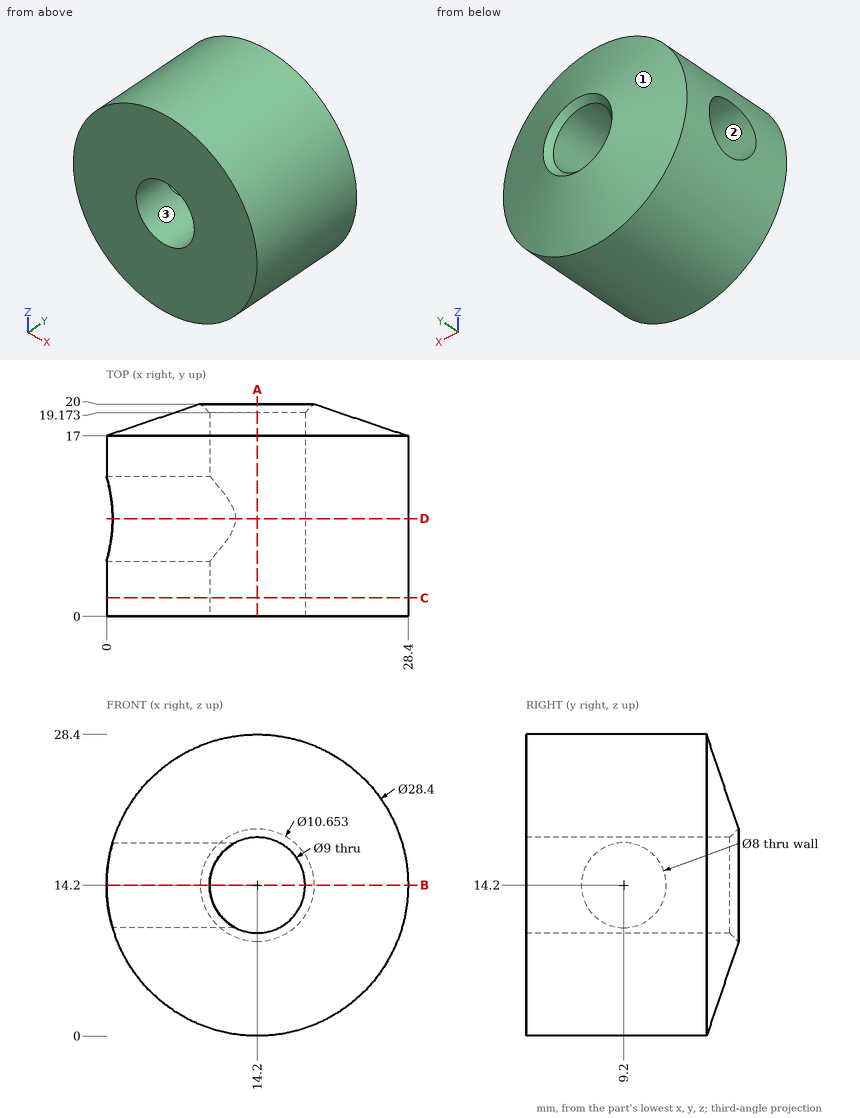
The figure shows three views and two pictorial views of one solid part (mm, origin at its lowest corner). Answer the questions. Round coordinates to 2 decimals unless told otherwise and drop trailing zeros. Write each loop counter-clockwise with the first axis right and the second up, starting at its lowest first coordinate (ties: lowest second). Pieces come first, ordered by that corner, then holes. Notation, with made-up numbers: (-8.75, 16) - (29.25, 16) arc R20 ccw to (29.25, 30) - close; hole circle Ø4 at (83, -24). An arc over 180 degrees is marked (long way). Use one line per item in the form item = value. Start each with the question number.
Item 1: Flat-ended cylindrical pins translate along their axes: pin 1 Ø10 at (y, z) = (8.5, 17.5) entering from -X; pin 2 Ø6 at (x, y) = (17.5, 6.5) entering from +Z; pin 3 Ø1 at (x, y) = (8.5, 2.5) entering from +Z; pin 4 Ø5 at (x, y) = (22, 17.5) entering from -Z. Find the tip coordinate at first contact, or state that the pin passes through.
Item 2: A cutting plane is placed at B-B (z = 14.2). Write down the section's boundary in (x, y).
Item 3: Find the intervals of material crossed by line 1 (X direction, y = 9.25, z = 14.2); line 2 (Z direction, x = 7.5, y = 8.5); line 3 (X direction, y = 14.25, z = 14.2), in increasing order. Write a range as [from, to].
Item 4: Determine the mould class of the marked faces 1, 2 and 3 for opening direction Y: +Y half, -Y half, draft (parallel to the pull), parting line (faces both ways), or undercut.
Item 5: A cutting plane is placed at D-D (y = 9.2). Write down the section's boundary in (x, z) (1 decimal).
Item 6: A cutting plane is placed at A-A (x = 14.2). Write down the section's boundary in (y, z), plus the area to 3 significant figures.
Item 7: A cutting plane is placed at C-C (y = 1.75). Write down the section's boundary in (x, z).
The answers:
q1.pin_1 = 0
q1.pin_2 = 28.4
q1.pin_3 = 27.41
q1.pin_4 = 1.05
q2.outline = (0, 0) - (9.7, 0) - (9.7, 5.2) - (0, 5.2) - close; (0, 13.2) - (9.7, 13.2) - (9.7, 19.17) - (8.87, 20) - (0, 17) - close; (18.7, 0) - (28.4, 0) - (28.4, 17) - (19.53, 20) - (18.7, 19.17) - close
q3.line_1 = [18.7, 28.4]
q3.line_2 = [1.68, 10.26], [18.14, 26.72]
q3.line_3 = [0, 9.7], [18.7, 28.4]
q4.face_1 = +Y half
q4.face_2 = undercut
q4.face_3 = draft
q5.outline = (0.6, 10.2) arc R14.2 ccw (long way) to (0.6, 18.2) - (12.1, 18.2) arc R4.5 cw (long way) to (12.1, 10.2) - close
q6.outline = (0, 0) - (17, 0) - (20, 8.87) - (19.17, 9.7) - (0, 9.7) - close; (0, 18.7) - (19.17, 18.7) - (20, 19.53) - (17, 28.4) - (0, 28.4) - close
q6.area = 361 mm^2
q7.outline = circle Ø28.4 at (14.2, 14.2); hole circle Ø9 at (14.2, 14.2)
